```python
from build123d import *

# Parameters (mm, degrees)
F1_DEPTH = 85
F0_R     = 10
F2_DEPTH = 3
F3_R     = 0.75
F4_DEPTH = 15
F5_START = 3
F5_DEPTH = 77


with BuildPart() as f1:
    # F0 (on Top) → F1 (new body)
    with BuildSketch(Plane.XY):
        with BuildLine():
            Line((-1.0081231615, -4.3175521048), (-1.0081231615, -5.9147009807))
            ThreePointArc((-1.0081231615, -5.9147009807), (-0.5058626868, -5.9786372145), (0, -6))
            Line((0, -6), (0, -4.3175521048))
            Line((0, -4.3175521048), (-1.0081231615, -4.3175521048))
        make_face()
        with BuildLine():
            ThreePointArc((0, -6), (0.5482317643, -5.9749009977), (1.0918768385, -5.8998139775))
            Line((1.0918768385, -5.8998139775), (1.0918768385, -4.3175521048))
            Line((1.0918768385, -4.3175521048), (0, -4.3175521048))
            Line((0, -4.3175521048), (0, -6))
        make_face()
        with BuildLine():
            ThreePointArc((1.0918768385, -5.8998139775), (4.6125514106, -3.8372346142), (6, 0))
            ThreePointArc((6, 0), (-3.8698359804, 4.5852338528), (-1.0081231615, -5.9147009807))
            Line((-1.0081231615, -5.9147009807), (-1.0081231615, -4.3175521048))
            Line((-1.0081231615, -4.3175521048), (0, -4.3175521048))
            Line((0, -4.3175521048), (1.0918768385, -4.3175521048))
            Line((1.0918768385, -4.3175521048), (1.0918768385, -5.8998139775))
        make_face()
    extrude(amount=F1_DEPTH)

    # F0 (on Top) → F2 (join)
    with BuildSketch(Plane.XY):
        Circle(F0_R)
        with BuildLine():
            ThreePointArc((-1.0081231615, -5.9147009807), (-3.8698359804, 4.5852338528), (6, 0))
            ThreePointArc((6, 0), (4.6125514106, -3.8372346142), (1.0918768385, -5.8998139775))
            ThreePointArc((1.0918768385, -5.8998139775), (0.5482317643, -5.9749009977), (0, -6))
            ThreePointArc((0, -6), (-0.5058626868, -5.9786372145), (-1.0081231615, -5.9147009807))
        make_face(mode=Mode.SUBTRACT)
    extrude(amount=F2_DEPTH)

    # F3 (on Right) → F4 (cut, symmetric)
    with BuildSketch(Plane.YZ):
        with Locations((0, 83.4703872204)):
            Circle(F3_R)
    extrude(amount=F4_DEPTH, both=True, mode=Mode.SUBTRACT)

    # F0 (on Top) → F5 (cut)
    with BuildSketch(Plane.XY.offset(F5_START)):
        with BuildLine():
            Line((-1.0081231615, -4.3175521048), (-1.0081231615, -5.9147009807))
            ThreePointArc((-1.0081231615, -5.9147009807), (-0.5058626868, -5.9786372145), (0, -6))
            Line((0, -6), (0, -4.3175521048))
            Line((0, -4.3175521048), (-1.0081231615, -4.3175521048))
        make_face()
        with BuildLine():
            ThreePointArc((0, -6), (0.5482317643, -5.9749009977), (1.0918768385, -5.8998139775))
            Line((1.0918768385, -5.8998139775), (1.0918768385, -4.3175521048))
            Line((1.0918768385, -4.3175521048), (0, -4.3175521048))
            Line((0, -4.3175521048), (0, -6))
        make_face()
    extrude(amount=F5_DEPTH, mode=Mode.SUBTRACT)


solid = f1.part
```
CAD build for the part. Positions are in the model's coordinates, mm. A direction names the side the tool comes from. Round coordinates to 2 decimals unless told otherwise and drop trailing zeros. Order: outer loops, then holes, each group sorted by start corner. A loop starts at its lowest first (then second) coordinate and runs counter-clockwise, first axis right, second up.
Q1. Slice it at D-D (z = 77). Write the cut outline in (x, y), and give its area (3 significant figures).
Q2. Which spindle directions (+Z, -Z, +X, -X, +Y, -Y) get a long thin tool onto all of the face, cutting with end or side? Do faces 1 (the flat face through (1.092, -5, 41)), 2 (the flat face through (0, 0, 0)). Say none if no direction does.
Q3. Drop flat-ended pins along their axis: pin 1 (8 mm diameter, centred on x = 2, z = 44, fed in from -Y); pin 2 (1.3 mm diameter, centred on y = -5, z = 32, fed in from +X); pin 3 (2 mm diameter, centred on x = 3, z = 34.5, fed in from +Y); pin 4 (1.4 mm diameter, centred on y = 0, z = 83.47, fed in from -X). Give the stop position or say it passes through.
Q4. Slice it at A-A (y = 0). Write the cut outline in (x, z).
Q5. Slice it at B-B (x = -3.75). Write the cut outline in (y, z).
Q6. Two-plate mould, pull along Z, no slides. Class faces 3 (the cylindrical face through (-2.17, -9.76, 1.48)), 4 (the flat face through (0, 0, 85)), 5 (the flat face through (0, -5, 80)): pulls with the +Z half, pulls with the -Z half, needs draft (parallel to the pull), parting line crosses it, or undercut.
Q7. Slice it at C-C (y = 8). Write the cut outline in (x, z), and give its area (3 significant figures).
Q8. Wall check: L1, parallel to Z at x = 3, y = 0; L2, parallel to Y at x = 0, z = 24; L3, parallel to Z at x = 7, y = 1.5. Give the ranges that are in metal, low to high.
Results below:
1. outline: (-1.01, -5.91) - (-1.01, -4.32) - (1.09, -4.32) - (1.09, -5.9) arc R6 ccw (long way) to start
1. area: 110 mm2
2. face 1: -Y
2. face 2: -Z, +X, -X, +Y, -Y
3. pin 1: stops at y = -5.91
3. pin 2: stops at x = 4.13
3. pin 3: stops at y = 5.66
3. pin 4: passes through
4. outline: (-10, 0) - (10, 0) - (10, 3) - (6, 3) - (6, 82.72) - (-6, 82.72) - (-6, 3) - (-10, 3) - close; (-6, 84.22) - (6, 84.22) - (6, 85) - (-6, 85) - close
5. outline: (-9.27, 0) - (9.27, 0) - (9.27, 3) - (4.68, 3) - (4.68, 85) - (-4.68, 85) - (-4.68, 3) - (-9.27, 3) - close; hole circle Ø1.5 at (0, 83.47)
6. face 3: needs draft
6. face 4: pulls with the +Z half
6. face 5: undercut
7. outline: (-6, 0) - (6, 0) - (6, 3) - (-6, 3) - close
7. area: 36.0 mm2
8. L1: z = 0 to 82.72, 84.22 to 85
8. L2: y = -4.32 to 6
8. L3: z = 0 to 3
